Verification items for the finished model (mm, model axes). Coordinates: 2 decimals unless noted, no trailing zeros. Write each loop counter-clockwise with the first axis right and the second up, starting at its lowest first coordinate (ties: lowest second). Pieces come first, ordered by that corner, then holes. Notation, with made-up numbers: M -21,22 L 28,22 A25 ccw 28,50 Z; hole C -37.5,52.5 d1. An arc over 180 degrees is marked long. Answer in a Markdown table with one row per item.
from build123d import *

# Parameters (mm, degrees)
SKETCH_1_W                   = 130
SKETCH_1_H                   = 16
EXTRUDE_1_DEPTH              = 7
HOLE_WIZARD_M5_1_D           = 5.8
HOLE_WIZARD_M5_1_CBORE_D     = 10
HOLE_WIZARD_M5_1_CBORE_DEPTH = 5
FILLET_1_R                   = 5
CUT_EXTRUDE_1_DEPTH          = 132.167831422


with BuildPart() as part:
    # 草图1 → 凸台-拉伸1 (new body)
    with BuildSketch(Plane.XY):
        with Locations((65, 8)):
            Rectangle(SKETCH_1_W, SKETCH_1_H)
    extrude(amount=EXTRUDE_1_DEPTH)

    # M5 六角凹头螺钉的柱形沉头孔1 (through all)
    with Locations(Plane(origin=(0, 0, 0), x_dir=(-1, 0, 0), z_dir=(0, 0, -1))):
        with Locations((-10, 8)):
            CounterBoreHole(HOLE_WIZARD_M5_1_D / 2, HOLE_WIZARD_M5_1_CBORE_D / 2, HOLE_WIZARD_M5_1_CBORE_DEPTH)

    # 圆角1
    fillet_1_edges = [part.edges().sort_by_distance(p)[0] for p in [
        (0, 16, 3.5),
        (0, 0, 3.5),
    ]]
    fillet(fillet_1_edges, radius=FILLET_1_R)

    # 草图4 → 切除-拉伸1 (cut, through all)
    with BuildSketch(Plane(origin=(0, 0, 0), x_dir=(-1, 0, 0), z_dir=(0, 0, -1))):
        with BuildLine():
            Line((-50, 5.2), (-120, 5.2))
            ThreePointArc((-120, 5.2), (-122.8, 8), (-120, 10.8))
            Line((-120, 10.8), (-50, 10.8))
            ThreePointArc((-50, 10.8), (-47.2, 8), (-50, 5.2))
        make_face()
    extrude(amount=-CUT_EXTRUDE_1_DEPTH, mode=Mode.SUBTRACT)


solid = part.part
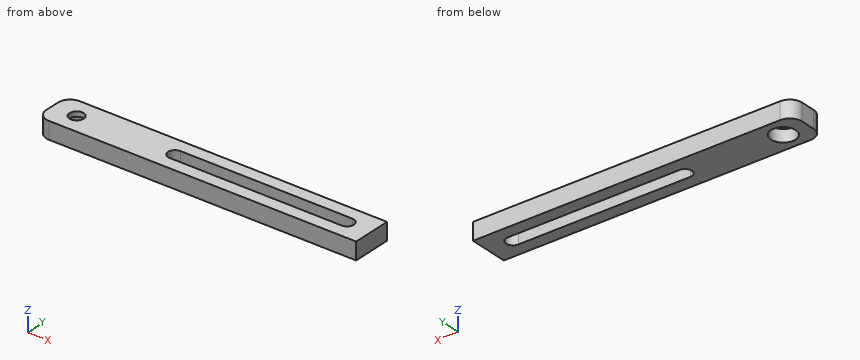
1) Sectioned sample at B-B (y = 8). Record the cut outline in (x, z).
Response values:
| item | result |
|---|---|
| outline | M 0,0 L 5,0 L 5,5 L 7.1,5 L 7.1,7 L 0,7 Z; M 12.9,5 L 15,5 L 15,0 L 47.2,0 L 47.2,7 L 12.9,7 Z; M 122.8,0 L 130,0 L 130,7 L 122.8,7 Z |
2) Sectioned sample at A-A (x = 10). Record the cut outline in (y, z).
Response values:
| item | result |
|---|---|
| outline | M 0,0 L 3,0 L 3,5 L 5.1,5 L 5.1,7 L 0,7 Z; M 10.9,5 L 13,5 L 13,0 L 16,0 L 16,7 L 10.9,7 Z |
3) Depth check by flat-ended pin: pin 1 (6 mm diameter, centred on x = 10, y = 8, fed in from -Z); pin 2 (5 mm diameter, centred on x = 10, y = 8, fed in from +Z); pin 3 (1.5 mm diameter, centred on x = 79, y = 4, fed in from -Z). Enter the tip coordinate at first touch or a pass-through.
Response values:
| item | result |
|---|---|
| pin 1 | stops at z = 5 |
| pin 2 | passes through |
| pin 3 | stops at z = 0 |
4) Sectioned sample at C-C (z = 2.5). Record the cut outline in (x, y), then the cut area to 3 significant figures.
Response values:
| item | result |
|---|---|
| outline | M 0,5 A5 ccw 5,0 L 130,0 L 130,16 L 5,16 A5 ccw 0,11 Z; hole C 10,8 d10; hole M 50,5.2 L 120,5.2 A2.8 ccw 120,10.8 L 50,10.8 A2.8 ccw Z |
| area | 1,570 mm² |
5) Thickness scan on L1, parallel to Y at x = 10, z = 3.1; L2, parallel to Y at x = 59.5, z = 5.75; L3, parallel to X at y = 9, z = 3.5. Record the ranges inside material, lowest first. Write a range as [from, to].
Response values:
| item | result |
|---|---|
| L1 | y = [0, 3], [13, 16] |
| L2 | y = [0, 5.2], [10.8, 16] |
| L3 | x = [0, 5.1], [14.9, 47.38], [122.62, 130] |
6) Sectioned sample at D-D (x = 101.5). Record the cut outline in (y, z).
Response values:
| item | result |
|---|---|
| outline | M 0,0 L 5.2,0 L 5.2,7 L 0,7 Z; M 10.8,0 L 16,0 L 16,7 L 10.8,7 Z |
